from build123d import *

# Parameters (mm, degrees)
ESBO_O1_W                    = 30
ESBO_O1_H                    = 60
RESSALTO_EXTRUS_O1_DEPTH     = 4.5
CORTE_EXTRUS_O2_DEPTH        = 63.010079826
CORTE_EXTRUS_O3_START        = -24.5
CORTE_EXTRUS_O3_DEPTH        = 24.5
ESBO_O4_W                    = 9
ESBO_O4_H                    = 24
RESSALTO_EXTRUS_O3_DEPTH     = 5
CHANFRO1_SIZE                = 6
CHANFRO1_SIZE_2              = 10.392304845
FILETE2_R                    = 5
CHANFRO1_OF_ESPELHAR2_SIZE   = 6
CHANFRO1_OF_ESPELHAR2_SIZE_2 = 10.392304845
FILETE3_R                    = 5
ESBO_O5_R                    = 2.75
CORTE_EXTRUS_O4_DEPTH        = 38.161808352
ESBO_O6_R                    = 4.5
ESBO_O6_R_2                  = 2.75
CORTE_EXTRUS_O5_DEPTH        = 4.5
ESBO_O7_R                    = 1.75
CORTE_EXTRUS_O6_DEPTH        = 38.161808352
ESPELHAR4_COPY_1_SKETCH_R    = 1.75
ESPELHAR4_COPY_1_DEPTH       = 38.161808352
CHANFRO2_SIZE                = 0.6


with BuildPart() as part:
    # Esboço1 → Ressalto-extrusão1 (new, symmetric)
    with BuildSketch(Plane.XY):
        Rectangle(ESBO_O1_W, ESBO_O1_H)
    extrude(amount=RESSALTO_EXTRUS_O1_DEPTH, both=True)

    # Esboço2 → Corte-extrusão2 (cut, through all)
    with BuildSketch(Plane.XZ.offset(30)):
        with BuildLine():
            Line((-5, 58.363424399), (-5, 4.5))
            ThreePointArc((-5, 4.5), (0, -0.5), (5, 4.5))
            Line((5, 4.5), (5, 58.363424399))
            Line((5, 58.363424399), (5, 166.090273197))
            Line((5, 166.090273197), (-5, 166.090273197))
            Line((-5, 166.090273197), (-5, 58.363424399))
        make_face()
    extrude(amount=-CORTE_EXTRUS_O2_DEPTH, mode=Mode.SUBTRACT)

    # Esboço3 → Corte-extrusão3 (cut)
    with BuildSketch(Plane(origin=(0, 27, 0), x_dir=(1, 0, 0), z_dir=(0, 1, 0)).offset(CORTE_EXTRUS_O3_START)):
        with BuildLine():
            ThreePointArc((-5, -4.5), (0, 0.5), (5, -4.5))
            Line((5, -4.5), (7.7, -4.5))
            ThreePointArc((7.7, -4.5), (0, 3.2), (-7.7, -4.5))
            Line((-7.7, -4.5), (-5, -4.5))
        make_face()
    corte_extrus_o3 = extrude(amount=CORTE_EXTRUS_O3_DEPTH, mode=Mode.SUBTRACT)

    # Espelhar1: Corte-extrusão3 across plane
    add(corte_extrus_o3.mirror(Plane.ZX), mode=Mode.SUBTRACT)

    # Esboço4 → Ressalto-extrusão3 (add)
    with BuildSketch(Plane(origin=(15, 0, 0), x_dir=(0, 0, -1), z_dir=(1, 0, 0))):
        Rectangle(ESBO_O4_W, ESBO_O4_H)
    ressalto_extrus_o3 = extrude(amount=RESSALTO_EXTRUS_O3_DEPTH)

    # Chanfro1
    # the kernel refuses this chamfer: 10.392304845, 6 mm, written as the material it takes off along each edge
    with BuildSketch(Plane(origin=(20, 12, -31.385783824), x_dir=(-0.9983227437537926, 0.05789386240267147, 0), z_dir=(0, 0, 1))) as chanfro1_piece_1_section:
        Polygon((CHANFRO1_SIZE * 0.998322743754, CHANFRO1_SIZE * 0.0578938624027), (-CHANFRO1_SIZE_2 * 0.057893862405, CHANFRO1_SIZE_2 * 0.998322743793), (0, 0), align=None)
    chanfro1_piece_1 = extrude(amount=62.771567647, mode=Mode.PRIVATE)
    chanfro1_piece_1 = split(chanfro1_piece_1, bisect_by=Plane(origin=(15, 8.382110688, 0), z_dir=(1, 0, 0)), keep=Keep.TOP, mode=Mode.PRIVATE)
    add(chanfro1_piece_1, mode=Mode.SUBTRACT)
    with BuildSketch(Plane(origin=(20, -12, 31.385783824), x_dir=(-0.9983227437537926, -0.05789386240267147, 0), z_dir=(0, 0, -1))) as chanfro1_piece_2_section:
        Polygon((CHANFRO1_SIZE * 0.998322743754, CHANFRO1_SIZE * 0.0578938624027), (-CHANFRO1_SIZE_2 * 0.057893862405, CHANFRO1_SIZE_2 * 0.998322743793), (0, 0), align=None)
    chanfro1_piece_2 = extrude(amount=62.771567647, mode=Mode.PRIVATE)
    chanfro1_piece_2 = split(chanfro1_piece_2, bisect_by=Plane(origin=(15, -8.382110688, 0), z_dir=(1, 0, 0)), keep=Keep.TOP, mode=Mode.PRIVATE)
    add(chanfro1_piece_2, mode=Mode.SUBTRACT)

    # Filete2
    filete2_edges = [part.edges().sort_by_distance(p)[0] for p in [
        (20, -1.607695155, 0),
        (20, 1.607695155, 0),
        (15, 10.267949192, 0),
        (15, -10.267949192, 0),
    ]]
    fillet(filete2_edges, radius=FILETE2_R)

    # Espelhar2: Ressalto-extrusão3 across plane
    add(ressalto_extrus_o3.mirror(Plane(origin=(0, 0, 0), x_dir=(0, 0, 1), z_dir=(1, 0, 0))))

    # Chanfro1 of Espelhar2
    # the kernel refuses this chamfer: 10.392304845, 6 mm, written as the material it takes off along each edge
    with BuildSketch(Plane(origin=(-20, 12, -31.385783824), x_dir=(0.9983227437537926, 0.05789386240267147, 0), z_dir=(0, 0, 1))) as chanfro1_of_espelhar2_piece_1_section:
        Polygon((CHANFRO1_OF_ESPELHAR2_SIZE * 0.998322743754, -CHANFRO1_OF_ESPELHAR2_SIZE * 0.0578938624027), (-CHANFRO1_OF_ESPELHAR2_SIZE_2 * 0.057893862405, -CHANFRO1_OF_ESPELHAR2_SIZE_2 * 0.998322743793), (0, 0), align=None)
    chanfro1_of_espelhar2_piece_1 = extrude(amount=62.771567647, mode=Mode.PRIVATE)
    chanfro1_of_espelhar2_piece_1 = split(chanfro1_of_espelhar2_piece_1, bisect_by=Plane(origin=(-15, 8.382110688, 0), z_dir=(-1, 0, 0)), keep=Keep.TOP, mode=Mode.PRIVATE)
    add(chanfro1_of_espelhar2_piece_1, mode=Mode.SUBTRACT)
    with BuildSketch(Plane(origin=(-20, -12, 31.385783824), x_dir=(0.9983227437537926, -0.05789386240267147, 0), z_dir=(0, 0, -1))) as chanfro1_of_espelhar2_piece_2_section:
        Polygon((CHANFRO1_OF_ESPELHAR2_SIZE * 0.998322743754, -CHANFRO1_OF_ESPELHAR2_SIZE * 0.0578938624027), (-CHANFRO1_OF_ESPELHAR2_SIZE_2 * 0.057893862405, -CHANFRO1_OF_ESPELHAR2_SIZE_2 * 0.998322743793), (0, 0), align=None)
    chanfro1_of_espelhar2_piece_2 = extrude(amount=62.771567647, mode=Mode.PRIVATE)
    chanfro1_of_espelhar2_piece_2 = split(chanfro1_of_espelhar2_piece_2, bisect_by=Plane(origin=(-15, -8.382110688, 0), z_dir=(-1, 0, 0)), keep=Keep.TOP, mode=Mode.PRIVATE)
    add(chanfro1_of_espelhar2_piece_2, mode=Mode.SUBTRACT)

    # Filete3
    filete3_edges = [part.edges().sort_by_distance(p)[0] for p in [
        (-20, -1.607695155, 0),
        (-20, 1.607695155, 0),
        (-15, 10.267949192, 0),
        (-15, -10.267949192, 0),
    ]]
    fillet(filete3_edges, radius=FILETE3_R)

    # Esboço5 → Corte-extrusão4 (cut, through all)
    with BuildSketch(Plane.XY.offset(4.5)):
        with Locations((15.5, 0)):
            Circle(ESBO_O5_R)
    corte_extrus_o4 = extrude(amount=-CORTE_EXTRUS_O4_DEPTH, mode=Mode.SUBTRACT)

    # Esboço6 → Corte-extrusão5 (cut)
    # profile 1 of 3: a face of its own
    with BuildSketch(Plane.XY.offset(4.5)):
        with BuildLine():
            Line((18.330127019, 4.5), (15.5, 4.5))
            ThreePointArc((15.5, 4.5), (18.681980515, 3.181980515), (20, 0))
            Line((20, 0), (20, 0.267949192))
            ThreePointArc((20, 0.267949192), (19.829629131, 1.562044418), (19.330127019, 2.767949192))
            Line((19.330127019, 2.767949192), (18.330127019, 4.5))
        make_face()
    # profile 2 of 3: a face of its own
    with BuildSketch(Plane.XY.offset(4.5)):
        with Locations((15.5, 0)):
            Circle(ESBO_O6_R)
        with Locations((15.5, 0)):
            Circle(ESBO_O6_R_2, mode=Mode.SUBTRACT)
    # profile 3 of 3: a face of its own
    with BuildSketch(Plane.XY.offset(4.5)):
        with BuildLine():
            Line((20, -0.267949192), (20, 0))
            ThreePointArc((20, 0), (18.681980515, -3.181980515), (15.5, -4.5))
            Line((15.5, -4.5), (18.330127019, -4.5))
            Line((18.330127019, -4.5), (19.330127019, -2.767949192))
            ThreePointArc((19.330127019, -2.767949192), (19.829629131, -1.562044418), (20, -0.267949192))
        make_face()
    corte_extrus_o5 = extrude(amount=-CORTE_EXTRUS_O5_DEPTH, mode=Mode.SUBTRACT)

    # Espelhar5: Corte-extrusão4, Corte-extrusão5 across plane
    add(corte_extrus_o4.mirror(Plane(origin=(0, 0, 0), x_dir=(0, 0, 1), z_dir=(1, 0, 0))), mode=Mode.SUBTRACT)
    add(corte_extrus_o5.mirror(Plane(origin=(0, 0, 0), x_dir=(0, 0, 1), z_dir=(1, 0, 0))), mode=Mode.SUBTRACT)

    # Esboço7 → Corte-extrusão6 (cut, through all)
    with BuildSketch(Plane.XY.offset(4.5)):
        with Locations((11.35, 14.75)):
            Circle(ESBO_O7_R)
    corte_extrus_o6 = extrude(amount=-CORTE_EXTRUS_O6_DEPTH, mode=Mode.SUBTRACT)

    # Espelhar3: Corte-extrusão6 across plane
    add(corte_extrus_o6.mirror(Plane.ZX), mode=Mode.SUBTRACT)

    # Espelhar4: Corte-extrusão6 across plane
    add(corte_extrus_o6.mirror(Plane(origin=(0, 0, 0), x_dir=(0, 0, 1), z_dir=(1, 0, 0))), mode=Mode.SUBTRACT)

    # Espelhar4 copy 1 sketch → Espelhar4 copy 1 (cut, through all)
    with BuildSketch(Plane(origin=(0, 0, 4.5), x_dir=(-1, 0, 0), z_dir=(0, 0, 1))):
        with Locations((11.35, 14.75)):
            Circle(ESPELHAR4_COPY_1_SKETCH_R)
    extrude(amount=-ESPELHAR4_COPY_1_DEPTH, mode=Mode.SUBTRACT)

    # Chanfro2
    chanfro2_edges = [part.edges().sort_by_distance(p)[0] for p in [
        (17.5, 5.937822174, -4.5),
        (17.5, -5.937822174, -4.5),
        (20, 0, -4.5),
        (19.829629131, -1.562044418, -4.5),
        (19.829629131, 1.562044418, -4.5),
        (15.170370869, 10.313599929, -4.5),
        (15.170370869, -10.313599929, -4.5),
        (-15, -20.803847577, -4.5),
        (-17.5, -5.937822174, -4.5),
        (-17.5, 5.937822174, -4.5),
        (-20, 0, -4.5),
        (-19.829629131, -1.562044418, -4.5),
        (-19.829629131, 1.562044418, -4.5),
        (-15.170370869, -10.313599929, -4.5),
        (-15.170370869, 10.313599929, -4.5),
        (-6.35, -2.5, 4.5),
        (0, -30, -4.5),
        (-15, 20.803847577, -4.5),
        (0, 30, -4.5),
        (15, -20.803847577, -4.5),
        (15, -30, 0),
        (-15, -30, 0),
        (-15, 30, 0),
        (15, 30, 0),
        (15, 20.803847577, -4.5),
    ]]
    chamfer(chanfro2_edges, length=CHANFRO2_SIZE)


solid = part.part
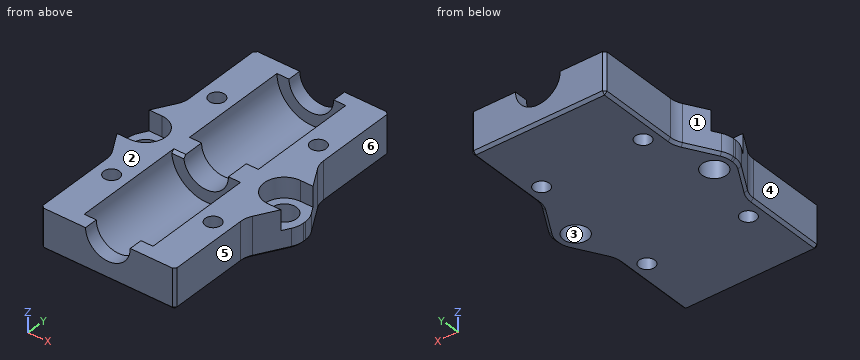
Input: part model. Units: mm. Frame: model coordinates. Face numbers are marked on the shaded views. A direction names the side the tool comes from. Coordinates: 2 decimals unless noted, no trailing zeros. Loops run counter-clockwise (first coordinate to the right, second up) from the corner with the lowest first, then second, coordinate; pieces in that order, holes last.
(1) Set-up query: the marked faces 4, 5 and 6. Return all of +Z, -Z, +X, -X, +Y, -Y with unobstructed straight access to the full face (end or side cutting, diameter ignored); none if empty.
(2) Pull-direction query (Y, two-part tool) for the marked faces 1, 2 and 3; classes: released by +Y, released by -Y, zero draft, split by the parting line, or undercut.
(3) Section D-D on x = -7. Return the cut outline in (y, z).
(4) Section B-B on y = -25. Return the cut outline in (x, z), then the cut area to 3 significant figures.
(5) Material intervals for probe 1 along Y at (x, z) = (-11.35, -0.5); probe 2 along Y at (x, z) = (-5, 1.75); probe 3 along X at (y, z) = (15, -4), sorted ascending.
(6) Section C-C on z = 2.25. Count the separate pieces of the cut face and the enclosed holes in it, then the cut area to 3 significant figures.
(7) Section A-A on y = -14.75. Return the cut outline in (x, z).
(8) First-contact query: pin 1 Ø2.5 at (y, z) = (23.5, 0) entering from +X; pin 2 Ø2 at (y, z) = (18, -2.5) entering from -X; pin 3 Ø0.8 at (x, z) = (17.5, 1.5) entering from -Y; pin 4 Ø4 at (x, z) = (1, 2) entering from +Y. Flat tips, straight axial feed; report the tip coordinate or a pass-through.
Data:
1. face 4: +Z, -Z, -X, -Y
1. face 5: +Z, -Z, +X, -Y
1. face 6: +Z, -Z, +X, +Y
2. face 1: released by +Y
2. face 2: zero draft
2. face 3: undercut
3. outline: (-30, -3.9) - (-29.4, -4.5) - (29.4, -4.5) - (30, -3.9) - (30, 4.5) - (27, 4.5) - (27, 1.29) - (2.5, 1.29) - (2.5, 4.5) - (-1.9, 4.5) - (-2.5, 3.9) - (-2.5, 1.29) - (-27, 1.29) - (-27, 4.5) - (-30, 4.5) - close
4. outline: (-15, -3.9) - (-14.4, -4.5) - (14.4, -4.5) - (15, -3.9) - (15, 4.5) - (7.7, 4.5) arc R7.7 cw to (-7.7, 4.5) - (-15, 4.5) - close
4. area: 177 mm2
5. probe 1: y = -30 to -16.5, -13 to 13, 16.5 to 30
5. probe 2: y = -30 to -27, -2.5 to 2.5, 27 to 30
5. probe 3: x = -14.9 to -13.08, -9.62 to 9.62, 13.08 to 14.9
6. separate pieces: 2
6. enclosed holes: 4
6. area: 925 mm2
7. outline: (-15, -3.9) - (-14.4, -4.5) - (-13.1, -4.5) - (-13.1, 4.5) - (-15, 4.5) - close; (-9.6, -4.5) - (9.6, -4.5) - (9.6, 4.5) - (7.7, 4.5) arc R7.7 cw to (-7.7, 4.5) - (-9.6, 4.5) - close; (13.1, -4.5) - (14.4, -4.5) - (15, -3.9) - (15, 4.5) - (13.1, 4.5) - close
8. pin 1: stops at x = 15
8. pin 2: stops at x = -15
8. pin 3: stops at y = -6.63
8. pin 4: passes through
